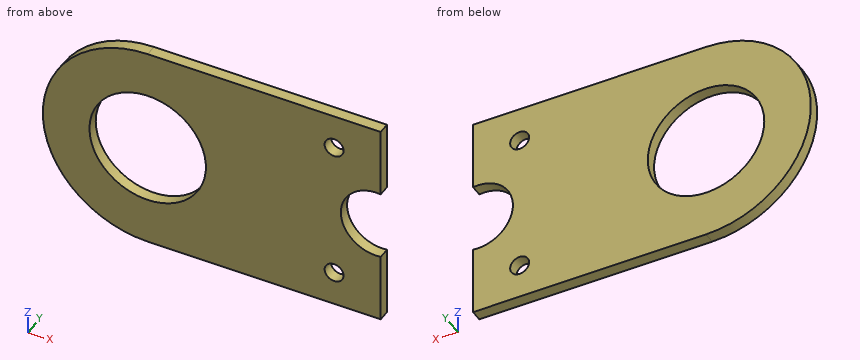
Autodesk Inventor part; units mm, degrees
ref_plane "YZ Plane" through (0, 0, 0) normal (1, 0, 0) x (0, 1, 0)
ref_plane "XZ Plane" through (0, 0, 0) normal (0, 1, 0) x (-1, 0, 0)
ref_plane "XY Plane" through (0, 0, 0) normal (0, 0, 1) x (1, 0, 0)
sketch "Sketch1" plane through (0, 0, 0) normal (0, 1, 0) x (-1, 0, 0)
  circle A0 centre (0, 0) radius 15.875
  arc A1 (0, -28.575) -> (0, 28.575) centre (0, 0) ccw
  line L0 (0, 28.575) -> (-63.5, 28.575)
  line L1 (-63.5, -28.575) -> (0, -28.575)
  line L2 (-36.1351, 28.575) -> (-36.1351, 9.525) construction
  line L3 (-36.1351, -28.575) -> (-36.1351, -9.525) construction
  line L4 (-63.5, 28.575) -> (-63.5, 9.525)
  line L5 (-63.5, -9.525) -> (-63.5, -28.575)
  line L6 (-63.5, 19.05) -> (-50.8, 19.05) construction
  line L7 (-63.5, -19.05) -> (-50.8, -19.05) construction
  arc A2 (-63.5, -9.525) -> (-63.5, 9.525) centre (-62.2343, 0) ccw
  circle A3 centre (-50.8, 19.05) radius 2.5797
  circle A4 centre (-50.8, -19.05) radius 2.5797
  dimension "d0" = 31.75
  dimension "d1" = 12.7
  dimension "d2" = 63.5
  dimension "d3" = 19.05
  dimension "d4" = 19.05
  dimension "d5" = 12.7
  dimension "d6" = 63.5
  dimension "d7" = 19.05
  dimension "d8" = 19.05
  dimension "d9" = 5.1594
  dimension "d10" = 5.1594
extrude "Extrusion1" add sketch "Sketch1" along normal blind 3.175
properties part number "motor extension"
Could you check a few things on this model? Use its own coordinates, in mm. Give positions to 0.01 mm unless a question says otherwise; leave off trailing zeros. Order: outer loops, then holes, each group sorted by start corner. A loop starts at its lowest first (then second) coordinate and runs counter-clockwise, first axis right, second up.
Q1. Suppose I cut it at B-B, the plane z = -7. Write out the boundary of the cut face in (x, y) (3 decimals).
Q2. I'm going to push flat-ended pins straight in: P1, Ø5, axis at x = 16, z = 10.5, coming from the -Y side; P2, Ø1.5, axis at x = -14, y = 1.5, coming from the +Z side. Where does each tip first touch, or does it pass through?
Q3. Suppose I cut it at A-A, the plane x = 50.8. Write out the boundary of the cut face in (y, z) (3 decimals).
Q4. If I drill on line 1 along Z through (x, y) = (50.8, 2.15) (3 decimals); line 2 along Z through (x, y) = (-0.5, 0.6); line 3 along Z through (x, y) = (49.5, 1.9) (3 decimals), over which ranges is the centre line in solid material (lowest first)?
Q5. Suppose I cut it at D-D, the plane z = 4.5. Write out the boundary of the cut face in (x, y) (3 decimals), and give its area (3 significant figures).
Q6. Suppose I cut it at C-C, the plane y = 0.8. Write out the boundary of the cut face in (x, z) (3 decimals).
Solution:
1. outline: (-27.704, 0) - (-14.248, 0) - (-14.248, 3.175) - (-27.704, 3.175) - close; (14.248, 0) - (55.652, 0) - (55.652, 3.175) - (14.248, 3.175) - close
2. P1: stops at y = 0
2. P2: stops at z = 25.32
3. outline: (0, -28.575) - (3.175, -28.575) - (3.175, -21.63) - (0, -21.63) - close; (0, -16.47) - (3.175, -16.47) - (3.175, 16.47) - (0, 16.47) - close; (0, 21.63) - (3.175, 21.63) - (3.175, 28.575) - (0, 28.575) - close
4. line 1: z = -28.575 to -21.63, -16.47 to 16.47, 21.63 to 28.575
4. line 2: z = -28.57 to -15.87, 15.87 to 28.57
4. line 3: z = -28.575 to -21.278, -16.822 to 16.822, 21.278 to 28.575
5. outline: (-28.218, 0) - (-15.224, 0) - (-15.224, 3.175) - (-28.218, 3.175) - close; (15.224, 0) - (53.744, 0) - (53.744, 3.175) - (15.224, 3.175) - close
5. area: 164 mm2
6. outline: (0, -28.575) - (63.5, -28.575) - (63.5, -9.525) arc R9.609 cw (long way) to (63.5, 9.525) - (63.5, 28.575) - (0, 28.575) arc R28.575 ccw to start; hole circle Ø31.75 at (0, 0); hole circle Ø5.159 at (50.8, -19.05); hole circle Ø5.159 at (50.8, 19.05)
